Check sheet for the modelled part. Datum: model origin and axes. Units: mm. Round coordinates to 2 decimals unless told otherwise and drop trailing zeros. Loops run counter-clockwise (first coordinate to the right, second up) from the corner with the lowest first, then second, coordinate; pieces in that order, holes last. Notation, with made-up numbers: (22, -8.5) -> (34, -8.5) arc R11 ccw to (34, -1.5) -> close; hole circle Ø5 at (83.5, 80). An arc over 180 degrees is marked (long way). One line per question, with ' | ' between items.
```python
from build123d import *

# Parameters (mm, degrees)
BOSS_EXTRU_1_DEPTH = 7
TROU_TARAUD_M41_D  = 3.3


with BuildPart() as part:
    # Esquisse1 → Boss.-Extru.1 (new body)
    with BuildSketch(Plane.XY):
        with BuildLine():
            Line((-15, 4), (0, 4))
            ThreePointArc((0, 4), (2.828427125, 2.828427125), (4, 0))
            Line((4, 0), (4, -5.5))
            ThreePointArc((4, -5.5), (2.29040669, -8.779334871), (-1.377018597, -9.255505264))
            Line((-1.377018597, -9.255505264), (-16.377018597, -3.755505264))
            ThreePointArc((-16.377018597, -3.755505264), (-18.938402027, 0.699277822), (-15, 4))
        make_face()
    extrude(amount=BOSS_EXTRU_1_DEPTH)

    # Trou taraudé M41 (through all)
    with Locations(Plane(origin=(0, 0, 0), x_dir=(1, 0, 0), z_dir=(0, 0, -1))):
        with Locations((-15, 0), (0, 0), (0, 5.5)):
            Hole(TROU_TARAUD_M41_D / 2)


solid = part.part
```
(1) Scan lines: probe 1 along Y at (x, z) = (0, 2); probe 2 along X at (y, z) = (0.25, 3.5); probe 3 along Y at (x, z) = (-14.75, 2.5). Record each from-to range of solid material in increasing order.
Answer:
probe 1: y = -9.5 to -7.15, -3.85 to -1.65, 1.65 to 4 | probe 2: x = -18.99 to -16.63, -13.37 to -1.63, 1.63 to 3.99 | probe 3: y = -4.35 to -1.63, 1.63 to 4
(2) Sectioned sample at C-C, the plane x = -5. Record the cut outline in (y, z).
Answer:
outline: (-7.93, 0) -> (4, 0) -> (4, 7) -> (-7.93, 7) -> close
(3) Go/stop test with flat-tipped pins: pin 1 (1 mm diameter, centred on y = -3, z = 2.5, fed in from -X); pin 2 (1.5 mm diameter, centred on x = -3.5, z = 1, fed in from -Y). Record where each tip stops, or that it passes through.
Answer:
pin 1: stops at x = -18.12 | pin 2: stops at y = -8.75
(4) Sectioned sample at D-D, the plane x = -9.25. Record the cut outline in (y, z), and give its area (3 significant figures).
Answer:
outline: (-6.37, 0) -> (4, 0) -> (4, 7) -> (-6.37, 7) -> close | area: 72.6 mm2
(5) Sectioned sample at B-B, the plane y = -5. Record the cut outline in (x, z).
Answer:
outline: (-12.98, 0) -> (-1.57, 0) -> (-1.57, 7) -> (-12.98, 7) -> close; (1.57, 0) -> (4, 0) -> (4, 7) -> (1.57, 7) -> close
(6) Mould release check, pull along X, two halves, no side actions. Record for faces 1 (the face through (-7, -1, 7)), 2 (the face through (0.4, -3.9, 3.5)), 3 (the face through (1.216, -1.115, 3.549)), 4 (the face through (-18.95, 0.62, 3.45)): +X half, -X half, draft (parallel to the pull), parting line (faces both ways), or undercut.
Answer:
face 1: draft | face 2: undercut | face 3: undercut | face 4: -X half
(7) Sectioned sample at A-A, the plane z = 6. Record the cut outline in (x, y), and give its area (3 significant figures).
Answer:
outline: (-16.38, -3.76) -> (-1.38, -9.26) arc R4 ccw to (4, -5.5) -> (4, 0) arc R4 ccw to (0, 4) -> (-15, 4) arc R4 ccw to start; hole circle Ø3.3 at (-15, 0); hole circle Ø3.3 at (0, -5.5); hole circle Ø3.3 at (0, 0) | area: 212 mm2
